Verification items for the finished model (mm, model axes). Face numbers are marked on the shaded views. A direction names the side the tool comes from. Coordinates: 2 decimals unless noted, no trailing zeros. Order: outer loops, then holes, each group sorted by start corner. A loop starts at its lowest first (then second) coordinate and runs counter-clockwise, first axis right, second up. Notation, with made-up numbers: (79, 76.5) -> (110, 76.5) arc R29 ccw to (110, 114.5) -> close; hole circle Ø1 at (56, -36.75). An arc over 180 degrees is marked (long way). Write each question's results on one line, items separated by ' | '. Start each with the question number.
(1) Draft check along X on the marked faces 1, 2 and 3. Enter one of: +X half, -X half, draft (parallel to the pull), parting line (faces both ways), or undercut.
(2) Go/stop test with flat-tipped pins: pin 1 (1 mm diameter, centred on x = 0.5, y = -2, fed in from +Z); pin 2 (1.5 mm diameter, centred on x = 3, z = 5.5, fed in from +Y); pin 3 (2 mm diameter, centred on x = 1.5, y = 0.5, fed in from +Z). Record where each tip stops, or that it passes through.
(3) Cross-section at A-A on y = 2.5. Enter the section's corners in (x, z).
(4) Set-up check for the marked faces 4, 5, 6, 7 and 8: record each of +Z, -Z, +X, -X, +Y, -Y from which the full face is reachable in a straight line by a thin tool's end or side.
(5) Cross-section at B-B on x = 2.5. Enter the section's corners in (y, z).
(6) Thickness scan on probe 1 along Y at (x, z) = (0.55, 1.25); probe 2 along Y at (x, z) = (3.05, 5.25). Record the ranges inside material, lowest first. Write a range as [from, to].
(7) Cross-section at D-D on z = 6.5. Enter the section's corners in (x, y).
```python
from build123d import *

# Parameters (mm, degrees)
ESQUISSE1_W        = 5
ESQUISSE1_H        = 5
BOSS_EXTRU_1_DEPTH = 5
ESQUISSE2_R        = 1
BOSS_EXTRU_2_DEPTH = 3.05
BOSS_EXTRU_3_START = 3.05
ESQUISSE3_R        = 1
BOSS_EXTRU_3_DEPTH = 3.05
ESQUISSE4_R        = 1
BOSS_EXTRU_4_DEPTH = 3.05
BOSS_EXTRU_5_START = 3.05
ESQUISSE5_R        = 1
BOSS_EXTRU_5_DEPTH = 3.05


with BuildPart() as part:
    # Esquisse1 → Boss.-Extru.1 (new body)
    with BuildSketch(Plane.XY):
        with Locations((2.5, 2.5)):
            Rectangle(ESQUISSE1_W, ESQUISSE1_H)
    extrude(amount=BOSS_EXTRU_1_DEPTH)

    # Esquisse2 → Boss.-Extru.2 (add)
    with BuildSketch(Plane(origin=(0, 5, 0), x_dir=(1, 0, 0), z_dir=(0, 1, 0))):
        with Locations(Location((2.5, -2.5, 0), (0, 0, 90))):
            Circle(ESQUISSE2_R)
    extrude(amount=BOSS_EXTRU_2_DEPTH)

    # Esquisse3 → Boss.-Extru.3 (add)
    with BuildSketch(Plane.XZ.offset(BOSS_EXTRU_3_START)):
        with Locations(Location((2.5, 2.5, 0), (0, 0, 270))):
            Circle(ESQUISSE3_R)
    extrude(amount=-BOSS_EXTRU_3_DEPTH)

    # Esquisse4 → Boss.-Extru.4 (add)
    with BuildSketch(Plane.XY.offset(5)):
        with Locations(Location((2.5, 2.5, 0), (0, 0, 180))):
            Circle(ESQUISSE4_R)
    extrude(amount=BOSS_EXTRU_4_DEPTH)

    # Esquisse5 → Boss.-Extru.5 (add)
    with BuildSketch(Plane(origin=(0, 0, 0), x_dir=(-1, 0, 0), z_dir=(0, 0, -1)).offset(BOSS_EXTRU_5_START)):
        with Locations((-2.5, 2.5)):
            Circle(ESQUISSE5_R)
    extrude(amount=-BOSS_EXTRU_5_DEPTH)


solid = part.part
```
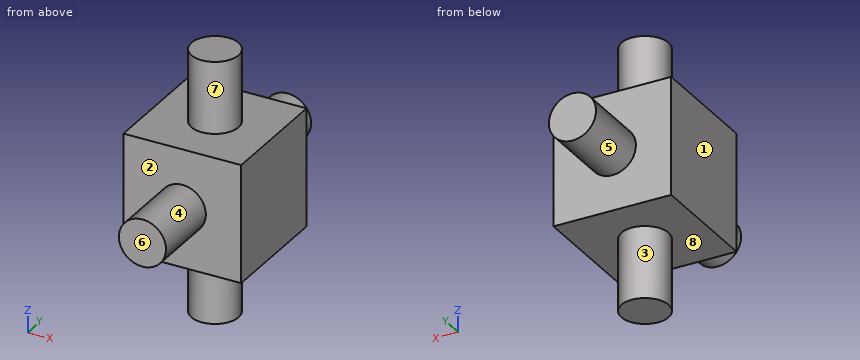
Results are:
1) face 1: -X half | face 2: draft | face 3: parting line
2) pin 1: passes through | pin 2: stops at y = 5 | pin 3: stops at z = 5
3) outline: (0, 0) -> (1.5, 0) -> (1.5, -3.05) -> (3.5, -3.05) -> (3.5, 0) -> (5, 0) -> (5, 5) -> (3.5, 5) -> (3.5, 8.05) -> (1.5, 8.05) -> (1.5, 5) -> (0, 5) -> close
4) face 4: -Y | face 5: +Y | face 6: +Z, -Z, +X, -X, -Y | face 7: +Z | face 8: -Z
5) outline: (-3.05, 1.5) -> (0, 1.5) -> (0, 0) -> (1.5, 0) -> (1.5, -3.05) -> (3.5, -3.05) -> (3.5, 0) -> (5, 0) -> (5, 1.5) -> (8.05, 1.5) -> (8.05, 3.5) -> (5, 3.5) -> (5, 5) -> (3.5, 5) -> (3.5, 8.05) -> (1.5, 8.05) -> (1.5, 5) -> (0, 5) -> (0, 3.5) -> (-3.05, 3.5) -> close
6) probe 1: y = [0, 5] | probe 2: y = [1.66, 3.34]
7) outline: circle Ø2 at (2.5, 2.5)
